```python
from build123d import *

# Parameters (mm, degrees)
SKETCH1_W                    = 150
SKETCH1_H                    = 40
BASE_FLANGE1_DEPTH           = 4
EDGE_FLANGE1_STRIP_W         = 24
EDGE_FLANGE1_STRIP_H         = 4
EDGE_FLANGE1_STRIP_CUT_DEPTH = 40
EDGE_FLANGE1_DEPTH           = 40
SKETCH9_R                    = 2
CUT_EXTRUDE1_DEPTH           = 10
FILLET1_R                    = 5
SKETCH10_R                   = 3.009837712
SKETCH10_R_2                 = 1.75
CUT_EXTRUDE2_DEPTH           = 10


# Sheet-metal steps are written as plain solids
with BuildPart() as part:
    # Sketch1 → Base-Flange1 (new body)
    with BuildSketch(Plane(origin=(0, 0, 0), x_dir=(1, 0, 0), z_dir=(0, 1, 0))):
        with Locations((75, 20)):
            Rectangle(SKETCH1_W, SKETCH1_H)
    extrude(amount=-BASE_FLANGE1_DEPTH)

    # Edge-Flange1 strip (across the edge) → Edge-Flange1 strip cut (cut)
    with BuildSketch(Plane(origin=(0, -4, 0), x_dir=(1, 0, 0), z_dir=(0, 0, -1))):
        with Locations((-8, -2)):
            Rectangle(EDGE_FLANGE1_STRIP_W, EDGE_FLANGE1_STRIP_H)
    extrude(amount=EDGE_FLANGE1_STRIP_CUT_DEPTH, mode=Mode.SUBTRACT)

    # Edge-Flange1 section (across the edge) → Edge-Flange1 (add)
    with BuildSketch(Plane(origin=(0, -4, 0), x_dir=(1, 0, 0), z_dir=(0, 0, -1))):
        with BuildLine():
            Line((-4, 4), (-4, 46))
            Line((-4, 46), (0, 46))
            Line((0, 46), (0, 4))
            ThreePointArc((0, 4), (1.171572875, 1.171572875), (4, 0))
            Line((4, 0), (4, -4))
            ThreePointArc((4, -4), (-1.656854249, -1.656854249), (-4, 4))
        make_face()
    extrude(amount=EDGE_FLANGE1_DEPTH)

    # Sketch9 → Cut-Extrude1 (cut)
    with BuildSketch(Plane(origin=(0, 0, 0), x_dir=(0, 0, -1), z_dir=(1, 0, 0))):
        with Locations(Location((7, -11, 0), (0, 0, 90))):
            Circle(SKETCH9_R)
        with Locations(Location((33, -43, 0), (0, 0, 90))):
            Circle(SKETCH9_R)
    extrude(amount=-CUT_EXTRUDE1_DEPTH, mode=Mode.SUBTRACT)

    # Fillet1
    fillet1_edges = [part.edges().sort_by_distance(p)[0] for p in [
        (-2, -50, 0),
        (-2, -50, -40),
        (150, -2, -40),
        (150, -2, 0),
    ]]
    fillet(fillet1_edges, radius=FILLET1_R)

    # Sketch10 → Cut-Extrude2 (cut)
    with BuildSketch(Plane(origin=(0, 0, 0), x_dir=(1, 0, 0), z_dir=(0, 1, 0))):
        with Locations(Location((102.263543229, 19.709585113, 0), (0, 0, 270))):
            Circle(SKETCH10_R)
        with Locations(Location((119.763543229, 19.709585113, 0), (0, 0, 270))):
            Circle(SKETCH10_R_2)
        with Locations(Location((84.763543229, 19.709585113, 0), (0, 0, 270))):
            Circle(SKETCH10_R_2)
    extrude(amount=-CUT_EXTRUDE2_DEPTH, mode=Mode.SUBTRACT)


solid = part.part
```
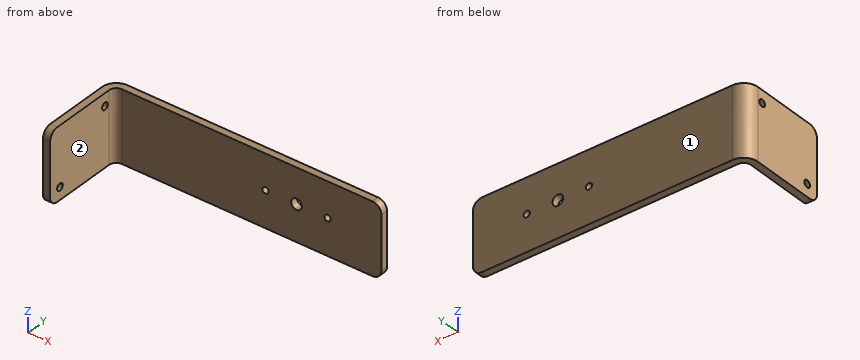
Here's how the part is built. I have some questions about the finished solid (model axes, mm). Face numbers are marked on the shaded views. A direction names the side the tool comes from. Coordinates: 2 decimals unless noted, no trailing zeros. Order: outer loops, then holes, each group sorted by start corner. A loop starts at its lowest first (then second) coordinate and runs counter-clockwise, first axis right, second up. Notation, with made-up numbers: (69.5, -27.75) -> (117.5, -27.75) arc R25 ccw to (117.5, 3.25) -> close; hole circle Ø7 at (58.5, -14.5). An arc over 180 degrees is marked (long way). Return JSON: item names as keys, results as strings.
1) If we section it at D-D on x = 20.5: List the corners of the cut face in (y, z) for me.
Conclusion:
{"outline": "(-4, -40) -> (0, -40) -> (0, 0) -> (-4, 0) -> close"}
2) If we section it at C-C on z = -28.5: List the corners of the cut face in (x, y) for me, plus the area to 3 significant figures.
Conclusion:
{"outline": "(-4, -50) -> (0, -50) -> (0, -8) arc R4 cw to (4, -4) -> (150, -4) -> (150, 0) -> (4, 0) arc R8 ccw to (-4, -8) -> close", "area": "790 mm²"}
3) If we section it at B-B on y = -11: List the corners of the cut face in (x, z) for me, plus the area to 3 significant figures.
Conclusion:
{"outline": "(-4, -40) -> (0, -40) -> (0, -9) -> (-4, -9) -> close; (-4, -5) -> (0, -5) -> (0, 0) -> (-4, 0) -> close", "area": "144 mm²"}
4) If I drill on probe 1 along Z at (x, y) = (-2.5, -43); probe 2 along X at (y, z) = (-33, -25.5), over which ranges is the centre line in solid material (lowest first)?
Conclusion:
{"probe 1": "z = -40 to -35, -31 to 0", "probe 2": "x = -4 to 0"}
5) I'm going to push flat-ended pins straight in: P1, Ø3, axis at y = -43, z = -33, coming from the +X side; P2, Ø12, axis at y = -17.5, z = -10.5, coming from the +X side; P3, Ø5.5, axis at x = 84.76, z = -19.71, coming from the -Y side. Where does each tip first touch, or does it pass through?
Conclusion:
{"P1": "passes through", "P2": "stops at x = 0", "P3": "stops at y = -4"}
6) On a 3-axis mill with a long thin cutter (end or side, diameter ignored), from which of +Z, -Z, +X, -X, +Y, -Y can I reach the whole of each face in a straight line? I mean the marked faces 1 and 2. Say none if no direction works.
Conclusion:
{"face 1": "+Z, -Z, +X, -X, +Y", "face 2": "+Z, -Z, +X, -Y"}
7) If we section it at A-A on z = -7: List the corners of the cut face in (x, y) for me, plus the area to 3 significant figures.
Conclusion:
{"outline": "(-4, -50) -> (0, -50) -> (0, -13) -> (-4, -13) -> close; (-4, -9) -> (0, -9) -> (0, -8) arc R4 cw to (4, -4) -> (150, -4) -> (150, 0) -> (4, 0) arc R8 ccw to (-4, -8) -> close", "area": "774 mm²"}
